from build123d import *

# Parameters (mm, degrees)
SKETCH_1_W          = 44
SKETCH_1_H          = 25
EXTRUDE_1_DEPTH     = 2
FILLET_1_RADIUS     = 12.5
FILLET_1_LENGTH     = 2
CUT_EXTRUDE_2_REACH = 27.382
SKETCH_3_R          = 4.1
SKETCH_3_R_2        = 1.5
SKETCH_4_W          = 25
SKETCH_4_H          = 2
EXTRUDE_2_DEPTH     = 20.5
CUT_EXTRUDE_3_REACH = 46.345
SKETCH_5_R          = 1.5
SKETCH_6_W          = 2
SKETCH_6_H          = 25
EXTRUDE_3_DEPTH     = 56
CUT_EXTRUDE_4_REACH = 88.328
SKETCH_7_R          = 4.1
SKETCH_7_R_2        = 1.5
FILLET_2_R          = 2


with BuildPart() as part:
    # 草图1 → 凸台-拉伸1 (new body)
    with BuildSketch(Plane(origin=(0, 0, 0), x_dir=(1, 0, 0), z_dir=(0, 1, 0))):
        Rectangle(SKETCH_1_W, SKETCH_1_H)
    extrude(amount=-EXTRUDE_1_DEPTH)

    # 圆角1: full round fillet: the end face becomes a half cylinder, R = half its width
    fillet_1_face = Plane((22, -1, 0), x_dir=(0, 1, 0), z_dir=(1, 0, 0))  # on the end face: x along it, z out of the body
    fillet_1_slab = fillet_1_face.offset(-FILLET_1_RADIUS / 2) * Box(FILLET_1_LENGTH, 2 * FILLET_1_RADIUS, FILLET_1_RADIUS, mode=Mode.PRIVATE)  # the body's end, R deep
    fillet_1_round = Plane((9.5, -1, 0), x_dir=(1, 0, 0), z_dir=(0, 1, 0)) * Cylinder(FILLET_1_RADIUS, FILLET_1_LENGTH, mode=Mode.PRIVATE)  # its axis R under the face
    add(fillet_1_slab - fillet_1_round, mode=Mode.SUBTRACT)

    # 草图3 → 切除-拉伸2 (cut, up to next)
    with BuildSketch(Plane(origin=(0, 0, 0), x_dir=(1, 0, 0), z_dir=(0, 1, 0)), mode=Mode.PRIVATE) as cut_extrude_2_sk1:
        with Locations(Location((9.5, 0, 0), (0, 0, 270))):
            Circle(SKETCH_3_R)
    cut_extrude_2_tool1 = extrude(cut_extrude_2_sk1.sketch, amount=-CUT_EXTRUDE_2_REACH, mode=Mode.PRIVATE) & part.part
    # 草图3 → 切除-拉伸2 (cut, up to next)
    with BuildSketch(Plane(origin=(0, 0, 0), x_dir=(1, 0, 0), z_dir=(0, 1, 0)), mode=Mode.PRIVATE) as cut_extrude_2_sk2:
        with Locations(Location((2.4, 0, 0), (0, 0, 270))):
            Circle(SKETCH_3_R_2)
    cut_extrude_2_tool2 = extrude(cut_extrude_2_sk2.sketch, amount=-CUT_EXTRUDE_2_REACH, mode=Mode.PRIVATE) & part.part
    # 草图3 → 切除-拉伸2 (cut, up to next)
    with BuildSketch(Plane(origin=(0, 0, 0), x_dir=(1, 0, 0), z_dir=(0, 1, 0)), mode=Mode.PRIVATE) as cut_extrude_2_sk3:
        with Locations(Location((9.5, 7.1, 0), (0, 0, 270))):
            Circle(SKETCH_3_R_2)
    cut_extrude_2_tool3 = extrude(cut_extrude_2_sk3.sketch, amount=-CUT_EXTRUDE_2_REACH, mode=Mode.PRIVATE) & part.part
    # 草图3 → 切除-拉伸2 (cut, up to next)
    with BuildSketch(Plane(origin=(0, 0, 0), x_dir=(1, 0, 0), z_dir=(0, 1, 0)), mode=Mode.PRIVATE) as cut_extrude_2_sk4:
        with Locations(Location((16.6, 0, 0), (0, 0, 270))):
            Circle(SKETCH_3_R_2)
    cut_extrude_2_tool4 = extrude(cut_extrude_2_sk4.sketch, amount=-CUT_EXTRUDE_2_REACH, mode=Mode.PRIVATE) & part.part
    # 草图3 → 切除-拉伸2 (cut, up to next)
    with BuildSketch(Plane(origin=(0, 0, 0), x_dir=(1, 0, 0), z_dir=(0, 1, 0)), mode=Mode.PRIVATE) as cut_extrude_2_sk5:
        with Locations(Location((9.5, -7.1, 0), (0, 0, 270))):
            Circle(SKETCH_3_R_2)
    cut_extrude_2_tool5 = extrude(cut_extrude_2_sk5.sketch, amount=-CUT_EXTRUDE_2_REACH, mode=Mode.PRIVATE) & part.part
    # 草图3 → 切除-拉伸2 (cut, up to next)
    with BuildSketch(Plane(origin=(0, 0, 0), x_dir=(1, 0, 0), z_dir=(0, 1, 0)), mode=Mode.PRIVATE) as cut_extrude_2_sk6:
        with Locations(Location((-9.2, 0, 0), (0, 0, 270))):
            Circle(SKETCH_3_R_2)
    cut_extrude_2_tool6 = extrude(cut_extrude_2_sk6.sketch, amount=-CUT_EXTRUDE_2_REACH, mode=Mode.PRIVATE) & part.part
    add(cut_extrude_2_tool1.solids().sort_by_distance((9.5, 0, 0))[0], mode=Mode.SUBTRACT)
    add(cut_extrude_2_tool2.solids().sort_by_distance((2.4, 0, 0))[0], mode=Mode.SUBTRACT)
    add(cut_extrude_2_tool3.solids().sort_by_distance((9.5, 0, -7.1))[0], mode=Mode.SUBTRACT)
    add(cut_extrude_2_tool4.solids().sort_by_distance((16.6, 0, 0))[0], mode=Mode.SUBTRACT)
    add(cut_extrude_2_tool5.solids().sort_by_distance((9.5, 0, 7.1))[0], mode=Mode.SUBTRACT)
    add(cut_extrude_2_tool6.solids().sort_by_distance((-9.2, 0, 0))[0], mode=Mode.SUBTRACT)

    # 草图4 → 凸台-拉伸2 (add)
    with BuildSketch(Plane.ZY.offset(22)):
        with Locations((0, -1)):
            Rectangle(SKETCH_4_W, SKETCH_4_H)
    extrude(amount=EXTRUDE_2_DEPTH)

    # 草图5 → 切除-拉伸3 (cut, up to next)
    with BuildSketch(Plane(origin=(0, 0, 0), x_dir=(1, 0, 0), z_dir=(0, 1, 0)), mode=Mode.PRIVATE) as cut_extrude_3_sk1:
        with Locations(Location((-26.2, 0, 0), (0, 0, 270))):
            Circle(SKETCH_5_R)
    cut_extrude_3_tool1 = extrude(cut_extrude_3_sk1.sketch, amount=-CUT_EXTRUDE_3_REACH, mode=Mode.PRIVATE) & part.part
    add(cut_extrude_3_tool1.solids().sort_by_distance((-26.2, 0, 0))[0], mode=Mode.SUBTRACT)

    # 草图6 → 凸台-拉伸3 (add)
    with BuildSketch(Plane(origin=(0, 0, 0), x_dir=(1, 0, 0), z_dir=(0, 1, 0))):
        with Locations((-41.5, 0)):
            Rectangle(SKETCH_6_W, SKETCH_6_H)
    extrude(amount=-EXTRUDE_3_DEPTH)

    # 草图7 → 切除-拉伸4 (cut, up to next)
    with BuildSketch(Plane.ZY.offset(42.5), mode=Mode.PRIVATE) as cut_extrude_4_sk1:
        with Locations((0, -28)):
            Circle(SKETCH_7_R)
    cut_extrude_4_tool1 = extrude(cut_extrude_4_sk1.sketch, amount=-CUT_EXTRUDE_4_REACH, mode=Mode.PRIVATE) & part.part
    # 草图7 → 切除-拉伸4 (cut, up to next)
    with BuildSketch(Plane.ZY.offset(42.5), mode=Mode.PRIVATE) as cut_extrude_4_sk2:
        with Locations((-7.1, -28)):
            Circle(SKETCH_7_R_2)
    cut_extrude_4_tool2 = extrude(cut_extrude_4_sk2.sketch, amount=-CUT_EXTRUDE_4_REACH, mode=Mode.PRIVATE) & part.part
    # 草图7 → 切除-拉伸4 (cut, up to next)
    with BuildSketch(Plane.ZY.offset(42.5), mode=Mode.PRIVATE) as cut_extrude_4_sk3:
        with Locations((0, -20.9)):
            Circle(SKETCH_7_R_2)
    cut_extrude_4_tool3 = extrude(cut_extrude_4_sk3.sketch, amount=-CUT_EXTRUDE_4_REACH, mode=Mode.PRIVATE) & part.part
    # 草图7 → 切除-拉伸4 (cut, up to next)
    with BuildSketch(Plane.ZY.offset(42.5), mode=Mode.PRIVATE) as cut_extrude_4_sk4:
        with Locations((7.1, -28)):
            Circle(SKETCH_7_R_2)
    cut_extrude_4_tool4 = extrude(cut_extrude_4_sk4.sketch, amount=-CUT_EXTRUDE_4_REACH, mode=Mode.PRIVATE) & part.part
    # 草图7 → 切除-拉伸4 (cut, up to next)
    with BuildSketch(Plane.ZY.offset(42.5), mode=Mode.PRIVATE) as cut_extrude_4_sk5:
        with Locations((0, -35.1)):
            Circle(SKETCH_7_R_2)
    cut_extrude_4_tool5 = extrude(cut_extrude_4_sk5.sketch, amount=-CUT_EXTRUDE_4_REACH, mode=Mode.PRIVATE) & part.part
    # 草图7 → 切除-拉伸4 (cut, up to next)
    with BuildSketch(Plane.ZY.offset(42.5), mode=Mode.PRIVATE) as cut_extrude_4_sk6:
        with Locations((0, -9.4)):
            Circle(SKETCH_7_R_2)
    cut_extrude_4_tool6 = extrude(cut_extrude_4_sk6.sketch, amount=-CUT_EXTRUDE_4_REACH, mode=Mode.PRIVATE) & part.part
    # 草图7 → 切除-拉伸4 (cut, up to next)
    with BuildSketch(Plane.ZY.offset(42.5), mode=Mode.PRIVATE) as cut_extrude_4_sk7:
        with Locations(Location((0, -46.6, 0), (0, 0, 180))):
            Circle(SKETCH_7_R_2)
    cut_extrude_4_tool7 = extrude(cut_extrude_4_sk7.sketch, amount=-CUT_EXTRUDE_4_REACH, mode=Mode.PRIVATE) & part.part
    add(cut_extrude_4_tool1.solids().sort_by_distance((-42.5, -28, 0))[0], mode=Mode.SUBTRACT)
    add(cut_extrude_4_tool2.solids().sort_by_distance((-42.5, -28, -7.1))[0], mode=Mode.SUBTRACT)
    add(cut_extrude_4_tool3.solids().sort_by_distance((-42.5, -20.9, 0))[0], mode=Mode.SUBTRACT)
    add(cut_extrude_4_tool4.solids().sort_by_distance((-42.5, -28, 7.1))[0], mode=Mode.SUBTRACT)
    add(cut_extrude_4_tool5.solids().sort_by_distance((-42.5, -35.1, 0))[0], mode=Mode.SUBTRACT)
    add(cut_extrude_4_tool6.solids().sort_by_distance((-42.5, -9.4, 0))[0], mode=Mode.SUBTRACT)
    add(cut_extrude_4_tool7.solids().sort_by_distance((-42.5, -46.6, 0))[0], mode=Mode.SUBTRACT)

    # 镜向1: part across plane


with BuildPart() as part_1:
    add(part.part)
    add(part.part.mirror(Plane.ZX.offset(-28)))

    # 圆角2
    fillet_2_edges = [part_1.edges().sort_by_distance(p)[0] for p in [
        (-42.5, 0, 0),
        (-42.5, -56, 0),
    ]]
    fillet(fillet_2_edges, radius=FILLET_2_R)


solid = part_1.part
Check sheet for the modelled part. Datum: model origin and axes. Units: mm. A direction names the side the tool comes from. Give positions to 0.01 mm unless a question says otherwise; leave off trailing zeros. Loops run counter-clockwise (first coordinate to the right, second up) from the corner with the lowest first, then second, coordinate; pieces in that order, holes last. Notation, with made-up numbers: M 82.25,40 L 106.25,40 A17 ccw 106.25,46 Z; hole C 11.5,15.5 d6. An arc over 180 degrees is marked long. Use a Markdown table: item, result. Add a question column.
Q1. Go/stop test with flat-tipped pins: pin 1 (5 mm diameter, centred on x = -9.2, z = 0, fed in from -Y); pin 2 (12.5 mm diameter, centred on y = -26.5, z = -0.5, fed in from +X); pin 3 (2.5 mm diameter, centred on y = -20.9, z = 0, fed in from +X). Record where each tip stops, or that it passes through.
Q2. Sectioned sample at B-B, the plane y = -9.4. Record the cut outline in (x, z).
Q3. Sectioned sample at C-C, the plane z = -7.1. Record the cut outline in (x, y), then the cut area to 3 significant figures.
Q4. Mould release check, pull along Z, two halves, no side actions. Record for faces 1 (the flat face through (-9, -2, 3)), 2 (the cylindrical face through (8.17, -55.01, -6.41)), 3 (the flat face through (-42, -28, 12.5)): pulls with the +Z half, pulls with the -Z half, needs draft (parallel to the pull), parting line crosses it, or undercut.
Q5. Tool access check on faces 4 (the flat face through (-9, -54, 3)), 5 (the cylindrical face through (5.86, -55.01, 1.89)). Record the directions out of +Z, -Z, +X, -X, +Y, -Y that give a thin tool (end or side, any length) a straight path to the whole face; none if there is none.
Q6. Sectioned sample at A-A, the plane x = -9.2. Record the cut outline in (y, z).
Q7. Sectioned sample at D-D, the plane y = -28. Record the cut outline in (x, z).
Q8. Scan lines: line 1 along Y through (x, z) = (-3.5, -11.25); line 2 along Y through (x, z) = (-41.75, 0); line 3 along X through (y, z) = (-0.65, 0). Record each from-to range of solid material in increasing order. Write a range as [from, to].
Verdict:
| question | item | result |
|---|---|---|
| 1 | pin 1 | y = -56 |
| 1 | pin 2 | x = -40.5 |
| 1 | pin 3 | through |
| 2 | outline | M -42.5,-12.5 L -40.5,-12.5 L -40.5,-1.5 L -42.5,-1.5 Z; M -42.5,1.5 L -40.5,1.5 L -40.5,12.5 L -42.5,12.5 Z |
| 3 | outline | M -42.5,-54 A2 ccw -40.5,-56 L 8,-56 L 8,-54 L -40.5,-54 L -40.5,-29.5 L -42.5,-29.5 Z; M -42.5,-26.5 L -40.5,-26.5 L -40.5,-2 L 8,-2 L 8,0 L -40.5,0 A2 ccw -42.5,-2 Z; M 11,-56 L 19.79,-56 L 19.79,-54 L 11,-54 Z; M 11,-2 L 19.79,-2 L 19.79,0 L 11,0 Z |
| 3 | area | 333 mm^2 |
| 4 | face 1 | needs draft |
| 4 | face 2 | undercut |
| 4 | face 3 | pulls with the +Z half |
| 5 | face 4 | +Z, -Z, +X |
| 5 | face 5 | +Y, -Y |
| 6 | outline | M -56,-12.5 L -54,-12.5 L -54,-1.5 L -56,-1.5 Z; M -56,1.5 L -54,1.5 L -54,12.5 L -56,12.5 Z; M -2,-12.5 L 0,-12.5 L 0,-1.5 L -2,-1.5 Z; M -2,1.5 L 0,1.5 L 0,12.5 L -2,12.5 Z |
| 7 | outline | M -42.5,-12.5 L -40.5,-12.5 L -40.5,-8.6 L -42.5,-8.6 Z; M -42.5,-5.6 L -40.5,-5.6 L -40.5,-4.1 L -42.5,-4.1 Z; M -42.5,4.1 L -40.5,4.1 L -40.5,5.6 L -42.5,5.6 Z; M -42.5,8.6 L -40.5,8.6 L -40.5,12.5 L -42.5,12.5 Z |
| 8 | line 1 | [-56, -54], [-2, 0] |
| 8 | line 2 | [-55.56, -48.1], [-45.1, -36.6], [-33.6, -32.1], [-23.9, -22.4], [-19.4, -10.9], [-7.9, -0.44] |
| 8 | line 3 | [-41.98, -27.7], [-24.7, -10.7], [-7.7, 0.9], [3.9, 5.4], [13.6, 15.1], [18.1, 22] |
